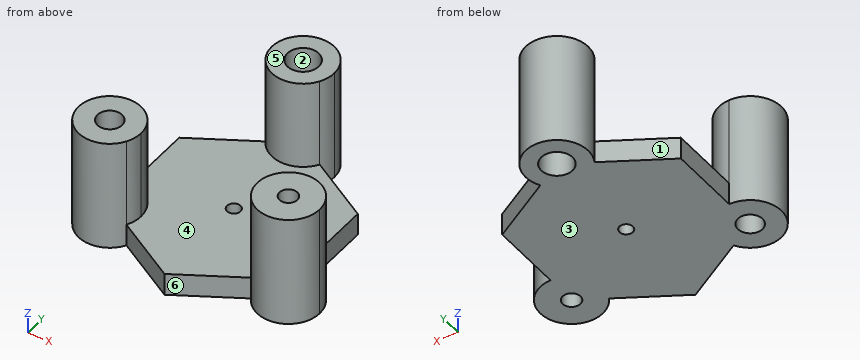
```python
from build123d import *

# Parameters (mm, degrees)
F1_DEPTH = 5
F2_DEPTH = 25
F3_D     = 7
F4_D     = 5.5
F5_D     = 4
F6_D     = 3


with BuildPart() as f1:
    # F0 (on Top) → F1 (new body)
    with BuildSketch(Plane.XY):
        with BuildLine():
            Line((20, -4.5470053838), (20, 11.5470053838))
            Line((20, 11.5470053838), (6.0621778265, 19.5940107676))
            ThreePointArc((6.0621778265, 19.5940107676), (0, 16.0940107676), (-6.0621778265, 19.5940107676))
            Line((-6.0621778265, 19.5940107676), (-20, 11.5470053838))
            Line((-20, 11.5470053838), (-20, -4.5470053838))
            ThreePointArc((-20, -4.5470053838), (-15.0502525317, -6.5972579155), (-13, -11.5470053838))
            ThreePointArc((-13, -11.5470053838), (-13.238519216, -13.3587386995), (-13.9378221735, -15.0470053838))
            Line((-13.9378221735, -15.0470053838), (0, -23.0940107676))
            Line((0, -23.0940107676), (13.9378221735, -15.0470053838))
            ThreePointArc((13.9378221735, -15.0470053838), (13.9378221735, -8.0470053838), (20, -4.5470053838))
        make_face()
    extrude(amount=F1_DEPTH)

    # F0 (on Top) → F2 (join)
    with BuildSketch(Plane.XY):
        with BuildLine():
            ThreePointArc((-20, -4.5470053838), (-26.0621778265, -15.0470053838), (-13.9378221735, -15.0470053838))
            Line((-13.9378221735, -15.0470053838), (-20, -11.5470053838))
            Line((-20, -11.5470053838), (-20, -4.5470053838))
        make_face()
        with BuildLine():
            Line((-20, -11.5470053838), (-13.9378221735, -15.0470053838))
            ThreePointArc((-13.9378221735, -15.0470053838), (-13.238519216, -13.3587386995), (-13, -11.5470053838))
            ThreePointArc((-13, -11.5470053838), (-15.0502525317, -6.5972579155), (-20, -4.5470053838))
            Line((-20, -4.5470053838), (-20, -11.5470053838))
        make_face()
        with BuildLine():
            Line((0, 23.0940107676), (6.0621778265, 19.5940107676))
            ThreePointArc((6.0621778265, 19.5940107676), (6.761480784, 21.2822774519), (7, 23.0940107676))
            ThreePointArc((7, 23.0940107676), (-1.8117333157, 29.8554915516), (-6.0621778265, 19.5940107676))
            Line((-6.0621778265, 19.5940107676), (0, 23.0940107676))
        make_face()
        with BuildLine():
            ThreePointArc((-6.0621778265, 19.5940107676), (0, 16.0940107676), (6.0621778265, 19.5940107676))
            Line((6.0621778265, 19.5940107676), (0, 23.0940107676))
            Line((0, 23.0940107676), (-6.0621778265, 19.5940107676))
        make_face()
        with BuildLine():
            ThreePointArc((27, -11.5470053838), (24.9497474683, -6.5972579155), (20, -4.5470053838))
            Line((20, -4.5470053838), (20, -11.5470053838))
            Line((20, -11.5470053838), (13.9378221735, -15.0470053838))
            ThreePointArc((13.9378221735, -15.0470053838), (21.8117333157, -18.3084861678), (27, -11.5470053838))
        make_face()
        with BuildLine():
            Line((20, -11.5470053838), (20, -4.5470053838))
            ThreePointArc((20, -4.5470053838), (13.9378221735, -8.0470053838), (13.9378221735, -15.0470053838))
            Line((13.9378221735, -15.0470053838), (20, -11.5470053838))
        make_face()
    extrude(amount=F2_DEPTH)

    # F3 (through all)
    with Locations(Plane(origin=(0, 0, 0), x_dir=(1, 0, 0), z_dir=(0, 0, -1))):
        with Locations((0, -23.0940107676)):
            Hole(F3_D / 2)

    # F4 (through all)
    with Locations(Plane(origin=(0, 0, 0), x_dir=(1, 0, 0), z_dir=(0, 0, -1))):
        with Locations((-20, 11.5470053838)):
            Hole(F4_D / 2)

    # F5 (through all)
    with Locations(Plane(origin=(0, 0, 0), x_dir=(1, 0, 0), z_dir=(0, 0, -1))):
        with Locations((20, 11.5470053838)):
            Hole(F5_D / 2)

    # F6 (through all)
    with Locations(Plane(origin=(0, 0, 0), x_dir=(1, 0, 0), z_dir=(0, 0, -1))):
        with Locations((0, 0)):
            Hole(F6_D / 2)


solid = f1.part
```
Work out the finished part from the listing and answer in its coordinate system (mm). Face numbers are marked on the shaded views. A direction names the side the tool comes from. Coordinates: 2 decimals unless noted, no trailing zeros. Order: outer loops, then holes, each group sorted by start corner. A loop starts at its lowest first (then second) coordinate and runs counter-clockwise, first axis right, second up. Notation, with made-up numbers: (50, 59.5) - (79, 59.5) arc R14 ccw to (79, 75.5) - close; hole circle Ø1 at (-19, -9.5). An arc over 180 degrees is marked (long way). Answer as a JSON object with one key per item and string values.
1. A tool of negligible diameter and unlimited length cuts with its end or side. For the marked faces 4, 5 and 6, from which of +Z, -Z, +X, -X, +Y, -Y can it reach the whole face along a straight path? Write none if from no direction.
Output values:
{"face 4": "+Z", "face 5": "+Z, +X, -X, +Y, -Y", "face 6": "+Z, -Z, -Y"}
2. Each of these flat-tipped pins is pushed along its axis until it touches: P1, Ø1.5, axis at y = 1.5, z = 3, coming from the -X side; P2, Ø10, axis at y = -6, z = 10, coming from the -X side; P3, Ø6, axis at x = 14, z = 12, coming from the -Y side. Where does it stop, or does it pass through?
Output values:
{"P1": "stops at x = -20", "P2": "stops at x = -26.98", "P3": "stops at y = -17.87"}
3. The mould has two halves that part along X. Classify the marked faces 1, 2 and 3: +X half, -X half, draft (parallel to the pull), parting line (faces both ways), or undercut.
Output values:
{"face 1": "-X half", "face 2": "undercut", "face 3": "draft"}
4. Consider line 1 (Y direction, x = 0, z = 11.75); line 2 (X direction, y = -16, z = 2); line 3 (Y direction, x = 20, z = 14.5). Determine where each line is inside the solid, lowest interval first.
Output values:
{"line 1": "y = 16.09 to 19.59, 26.59 to 30.09", "line 2": "x = -25.4 to -14.6, -12.29 to 12.29, 14.6 to 25.4", "line 3": "y = -18.55 to -13.55, -9.55 to -4.55"}
5. Find section B-B on y = 0. Determine the outline of the cut face in (x, z), plus the area to 3 significant figures.
Output values:
{"outline": "(-20, 0) - (-1.5, 0) - (-1.5, 5) - (-20, 5) - close; (1.5, 0) - (20, 0) - (20, 5) - (1.5, 5) - close", "area": "185 mm²"}
6. Find section C-C on x = -22. Determine the outline of the cut face in (y, z), plus the area to 3 significant figures.
Output values:
{"outline": "(-18.26, 0) - (-13.43, 0) - (-13.43, 25) - (-18.26, 25) - close; (-9.66, 0) - (-4.84, 0) - (-4.84, 25) - (-9.66, 25) - close", "area": "241 mm²"}
7. Find section A-A on z = 20.5. Determine the outline of the cut face in (x, y), plus the area to 3 significant figures.
Output values:
{"outline": "circle Ø14 at (-20, -11.55); circle Ø14 at (0, 23.09); circle Ø14 at (20, -11.55); hole circle Ø5.5 at (-20, -11.55); hole circle Ø7 at (0, 23.09); hole circle Ø4 at (20, -11.55)", "area": "387 mm²"}
8. Find section D-D on y = 8. Determine the outline of the cut face in (x, z), plus the area to 3 significant figures.
Output values:
{"outline": "(-20, 0) - (20, 0) - (20, 5) - (-20, 5) - close", "area": "200 mm²"}
